```python
from build123d import *

# Parameters (mm, degrees)
SKETCH1_W                   = 127
SKETCH1_H                   = 96.52
BOSS_EXTRUDE1_DEPTH         = 15.875
SKETCH2_W                   = 127
SKETCH2_H                   = 96.52
SKETCH2_R                   = 15.875
CUT_EXTRUDE1_DEPTH          = 3.175
F_1_4_0_25_DIAMETER_HOLE1_D = 6.35


with BuildPart() as part:
    # Sketch1 → Boss-Extrude1 (new body)
    with BuildSketch(Plane(origin=(0, 0, 0), x_dir=(1, 0, 0), z_dir=(0, 1, 0))):
        Rectangle(SKETCH1_W, SKETCH1_H)
    extrude(amount=BOSS_EXTRUDE1_DEPTH)

    # Sketch2 → Cut-Extrude1 (cut)
    with BuildSketch(Plane(origin=(0, 15.875, 0), x_dir=(1, 0, 0), z_dir=(0, 1, 0))):
        Rectangle(SKETCH2_W, SKETCH2_H)
        with Locations(Location((0, -8.89, 0), (0, 0, 270))):
            Circle(SKETCH2_R, mode=Mode.SUBTRACT)
    extrude(amount=-CUT_EXTRUDE1_DEPTH, mode=Mode.SUBTRACT)

    # 1/4 (0.25) Diameter Hole1 (through all)
    with Locations(Plane(origin=(0, 12.7, 0), x_dir=(1, 0, 0), z_dir=(0, 1, 0))):
        with Locations((15.24, -29.21), (0, -37.465), (0, 16.51), (-15.24, -29.21)):
            Hole(F_1_4_0_25_DIAMETER_HOLE1_D / 2)


solid = part.part
```
Here's how the part is built. I have some questions about the finished solid (model axes, mm). A direction names the side the tool comes from. Coordinates: 2 decimals unless noted, no trailing zeros. Order: outer loops, then holes, each group sorted by start corner. A loop starts at its lowest first (then second) coordinate and runs counter-clockwise, first axis right, second up. Notation, with made-up numbers: (50.5, -17) - (73.5, -17) arc R29 ccw to (73.5, 3) - close; hole circle Ø2 at (-36.75, 63). An arc over 180 degrees is marked (long way). One line per question, with ' | ' between items.
(1) Suppose I cut it at C-C on z = 8.89. List the corners of the cut face in (x, y) for me (3 decimals), and give its area (3 significant figures).
Report:
outline: (-63.5, 0) - (63.5, 0) - (63.5, 12.7) - (15.875, 12.7) - (15.875, 15.875) - (-15.875, 15.875) - (-15.875, 12.7) - (-63.5, 12.7) - close | area: 1,710 mm2
(2) If I drill on L1, parallel to Z at x = 0, y = 10.25 (3 decimals); L2, parallel to X at y = 7.25, z = 29.21 (3 decimals); L3, parallel to Z at x = -15.24, y = 4.5 (3 decimals), over which ranges is the centre line in solid material (lowest first)?
Report:
L1: z = -48.26 to -19.685, -13.335 to 34.29, 40.64 to 48.26 | L2: x = -63.5 to -18.415, -12.065 to 12.065, 18.415 to 63.5 | L3: z = -48.26 to 26.035, 32.385 to 48.26
(3) Suppose I cut it at D-D on x = -46. List the corners of the cut face in (y, z) for me.
Report:
outline: (0, -48.26) - (12.7, -48.26) - (12.7, 48.26) - (0, 48.26) - close
(4) Will this pin go through, and if not, where does the flat tip stop? pin 1 (1 mm diameter, centred on x = -7.5, z = -19, fed in from +Y).
Report:
pin 1: stops at y = 12.7
(5) For faces 1 (the cylindrical face through (-14.55, 6.26, 32.31)), 2 (the cylindrical face through (-9.66, 14.31, -3.71)), which set-ups out of +Z, -Z, +X, -X, +Y, -Y let a thin tool reach every point of the face, with its end or its side?
Report:
face 1: +Y, -Y | face 2: +Y
(6) If we mould it in two halves opening along Z, with no side actions, what happens to faces 3 (the cylindrical face through (15.93, 6.26, 32.31)), 4 (the flat face through (-1, 0, -1)), 5 (the flat face through (-1, 6, 48.26))? For each: pulls with the +Z half, pulls with the -Z half, needs draft (parallel to the pull), parting line crosses it, or undercut.
Report:
face 3: undercut | face 4: needs draft | face 5: pulls with the +Z half
(7) Suppose I cut it at A-A on z = 29.21. List the corners of the cut face in (x, y) for me (3 decimals).
Report:
outline: (-63.5, 0) - (-18.415, 0) - (-18.415, 12.7) - (-63.5, 12.7) - close; (-12.065, 0) - (12.065, 0) - (12.065, 12.7) - (-12.065, 12.7) - close; (18.415, 0) - (63.5, 0) - (63.5, 12.7) - (18.415, 12.7) - close
(8) Suppose I cut it at B-B on z = -16.51. List the corners of the cut face in (x, y) for me (3 decimals).
Report:
outline: (-63.5, 0) - (-3.175, 0) - (-3.175, 12.7) - (-63.5, 12.7) - close; (3.175, 0) - (63.5, 0) - (63.5, 12.7) - (3.175, 12.7) - close
